The listing builds one solid part. Answer for the finished solid, in the listing's coordinates (mm). Face numbers are marked on the shaded views. A direction names the side the tool comes from. Round coordinates to 2 decimals unless told otherwise and drop trailing zeros. Loops run counter-clockwise (first coordinate to the right, second up) from the corner with the lowest first, then second, coordinate; pieces in that order, holes last. Notation, with made-up numbers: (-5, 12.5) -> (3, 12.5) arc R17 cw to (3, 16.5) -> close; hole circle Ø3 at (87.25, 28.5). An arc over 180 degrees is marked (long way). Use a Markdown table: item, result. Add a question column.
Q1. Which of the six approach directions +Z, -Z, +X, -X, +Y, -Y give full straight-line access (tool end or side, diameter ignored) to the marked faces 1, 2 and 3?
Q2. For a pull along Y with two mould halves and no side action, classify the marked faces 4, 5 and 6 as released by +Y, released by -Y, zero draft, split by the parting line, or undercut.
Q3. Given pin 1 Ø4 at (x, z) = (0, 88.9) entering from +Y; pin 2 Ø1.5 at (x, z) = (18.5, 86.5) entering from -Y; pin 3 Ø23 at (x, y) = (-2, -11.5) entering from +Z; pin 4 Ø1 at (x, y) = (21, 29) entering from -Z, each flat-ended and moving along its own axis, determine where each tip first touches the part or whether it passes through.
Q4. Section D-D on z = 14 is taken. Give the vertices of the cut face in (x, y), then the cut area to 3 significant figures.
Q5. Section B-B on z = 88.5 is taken. Give the vertices of the cut face in (x, y) (3 decimals).
Q6. Consider line 1 (Y direction, x = 0, z = 24); line 2 (Y direction, x = -13, z = 72.5); line 3 (Z direction, x = 0, y = 30) (3 decimals). Determine where each line is inside the solid, lowest interval first.
Q7. Section C-C on y = -19 is taken. Give the vertices of the cut face in (x, z), then the cut area to 3 significant figures.
Autodesk Fusion 360 part; units mm, degrees
sketch "Sketch8" plane through (0, 0, 0) normal (0, 0, 1) x (1, 0, 0)
  circle A0 centre (0, 0) radius 37.3062
  circle A1 centre (0, 0) radius 27.7812
  dimension "d25" = 74.6125
  dimension "d26" = 55.5625
extrude "Extrude4" add sketch "Sketch8" along normal blind 50.8
sketch "Sketch9" plane through (0, 0, 50.8) normal (0, 0, 1) x (-1, 0, 0)
  circle A0 centre (0, 0) radius 27.7812
  circle A1 centre (0, 0) radius 37.3062
  circle A2 centre (0, 0) radius 37.3062
  circle A3 centre (0, 0) radius 9.9219
  line L0 (0, 0) -> (-27.7812, 0)
  line L1 (0, 0) -> (27.7812, 0)
  dimension "d29" = 19.8438
extrude "Extrude5" add sketch "Sketch9" along normal blind 6.35 contours A0 A3 L0 L1 | A1 A2 picked at (-14.6242, 16.1245)
sketch "Sketch10" plane through (0, 0, 57.15) normal (0, 0, 1) x (-1, 0, 0)
  arc A0 (9.9219, 0) -> (-9.9219, 0) centre (0, 0) ccw
  line L0 (9.9219, 0) -> (27.7812, 0)
  arc A1 (-27.7812, 0) -> (27.7812, 0) centre (0, 0) ccw
  line L1 (-27.7812, 0) -> (-9.9219, 0)
  circle A2 centre (0, 0) radius 37.3062
  line L2 (0, 0) -> (0, 9.9219)
  circle A3 centre (0, 9.9219) radius 19.05
  circle A4 centre (0, 9.9219) radius 22.225
  circle A5 centre (0, 0) radius 32.1469
  circle A6 centre (0, 0) radius 37.3062
  circle A7 centre (0, 0) radius 27.7812
  line L3 (27.7812, 0) -> (19.8874, 0)
  line L4 (-19.8874, 0) -> (-27.7812, 0)
  dimension "d32" = 38.1
  dimension "d33" = 44.45
extrude "Extrude6" add sketch "Sketch10" along normal blind 50.8 contours L0 A3 A4 A7 | L0 L1 A3 A4 | L0 A4 A7 L3 | L1 A3 A4 A7 | A5 | L1 A4 A7 L4 | A3 A4 A7 | A2 A6
ref_plane "WorkPlane1" through (0, -38.1, 0) normal (0, 1, 0) x (0, 0, 1)
sketch "Sketch11" plane through (0, -38.1, 0) normal (0, 1, 0) x (1, 0, 0)
  line L0 (0, 0) -> (0, -88.9)
  circle A0 centre (0, -88.9) radius 3.175
  dimension "d37" = 6.35
hole "Hole2" at (0, -38.1, 88.9) direction (0, -1, 0) diameter 6.35 depth 15.24 tip angle 118
ref_plane "WorkPlane2" through (0, 38.1, 0) normal (0, 1, 0) x (0, 0, 1)
sketch "Sketch12" plane through (0, 38.1, 0) normal (0, 1, 0) x (1, 0, 0)
  line L0 (0, 0) -> (0, -88.9)
  circle A0 centre (0, -88.9) radius 3.175
  line L1 (0, -88.9) -> (0, -107.95)
  dimension "d42" = 88.9
  dimension "d43" = 6.35
  dimension "d47" = 19.05
hole "Hole3" at (0, 38.1, 88.9) direction (0, -1, 0) diameter 6.35 depth 15.24 tip angle 118
sketch "Sketch7" plane through (0, 0, 0) normal (0, 0, 1) x (1, 0, 0)
equation "d25 = 3 in - ( ( 1 / 16 ) * 1 in )"
equation "d26 = 3 in - ( ( 1 / 16 ) * 1 in ) - ( ( 3 / 4 ) * 1 in )"
equation "d29 = ( ( 3 / 4 ) * 1 in ) + ( 1 / 32 ) * 1 in"
equation "d33 = 1.5 in + ( ( 1 / 4 ) * 1 in )"
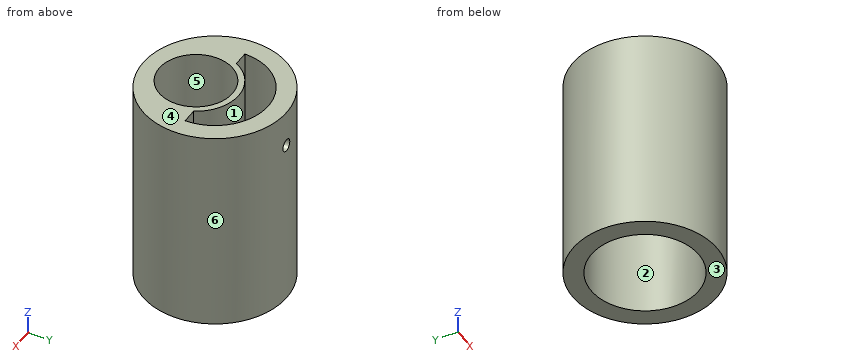
Checked values:
| question | item | result |
|---|---|---|
| 1 | face 1 | +Z, -Z |
| 1 | face 2 | -Z |
| 1 | face 3 | -Z, +X, -X, +Y, -Y |
| 2 | face 4 | zero draft |
| 2 | face 5 | undercut |
| 2 | face 6 | split by the parting line |
| 3 | pin 1 | stops at y = 12.3 |
| 3 | pin 2 | stops at y = -32.81 |
| 3 | pin 3 | stops at z = 57.15 |
| 3 | pin 4 | stops at z = 0 |
| 4 | outline | circle Ø74.61 at (0, 0); hole circle Ø55.56 at (0, 0) |
| 4 | area | 1,950 mm2 |
| 5 | outline | (-27.781, 0) arc R27.781 cw to (-3.15, 27.602) -> (-3.15, 37.173) arc R37.306 ccw (long way) to (3.15, 37.173) -> (3.15, 27.602) arc R27.781 cw to (27.781, 0) -> (19.887, 0) arc R22.225 ccw to (-19.887, 0) -> close; hole circle Ø38.1 at (0, -9.922) |
| 6 | line 1 | y = -37.31 to -27.78, 27.78 to 37.31 |
| 6 | line 2 | y = -34.97 to -23.85, 4 to 8.1, 24.55 to 34.97 |
| 6 | line 3 | z = 0 to 85.725, 92.075 to 107.95 |
| 7 | outline | (-32.11, 0) -> (-20.27, 0) -> (-20.27, 50.8) -> (20.27, 50.8) -> (20.27, 0) -> (32.11, 0) -> (32.11, 107.95) -> (16.75, 107.95) -> (16.75, 57.15) -> (-16.75, 57.15) -> (-16.75, 107.95) -> (-32.11, 107.95) -> close |
| 7 | area | 3,170 mm2 |
